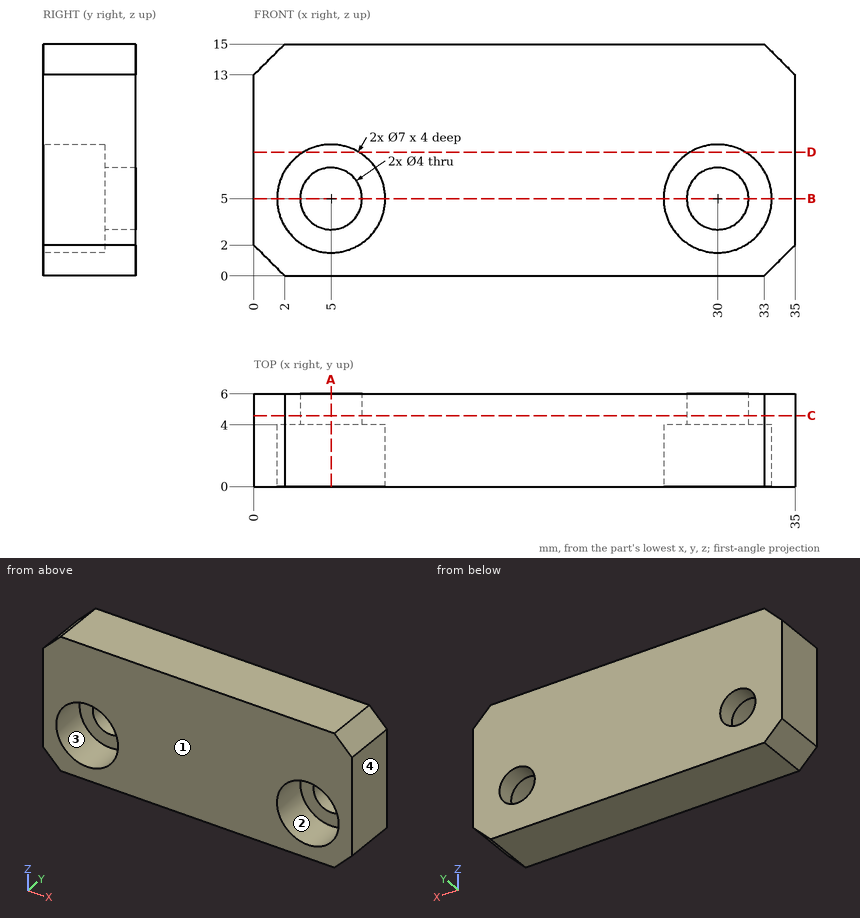
Could you check a few things on this drawing? It's one solid part, dimensions in mm from its lowest x, y, z. Coordinates: 2 decimals unless noted, no trailing zeros. Order: outer loops, then holes, each group sorted by start corner. A loop starts at its lowest first (then second) coordinate and runs counter-clockwise, first axis right, second up.
1. If we section it at C-C (y = 4.6): Please give me the cut outline in (x, z), then the cut area to 3 significant figures.
2. I need wall thicknesses on line 1 (X direction, y = 2.2, z = 4.5); line 2 (Z direction, x = 5, y = 1.15); line 3 (Z direction, x = 30, y = 4.85). Which ranges of each line are inside material? Lowest first, please.
3. If we section it at D-D (z = 8): Please give me the cut outline in (x, y), then the cut area to 3 significant figures.
4. If we section it at A-A (x = 5): Please give me the cut outline in (y, z).
5. If we section it at B-B (z = 5): Please give me the cut outline in (x, y).
6. Thinking about a two-plate mould opening in X: for the marked faces 1, 2, 3 and 4, which applies, +X half, -X half, draft (parallel to the pull), parting line (faces both ways), or undercut?
7. I'm going to push flat-ended pins straight in: pin 1 (5.5 mm diameter, centred on x = 30, z = 5, fed in from -Y); pin 2 (7.5 mm diameter, centred on x = 5, z = 4, fed in from -Y); pin 3 (3.5 mm diameter, centred on x = 5, z = 5, fed in from +Y). Where does each tip first touch, or does it pass through?
Entries:
1. outline: (0, 2) - (2, 0) - (33, 0) - (35, 2) - (35, 13) - (33, 15) - (2, 15) - (0, 13) - close; hole circle Ø4 at (5, 5); hole circle Ø4 at (30, 5)
1. area: 492 mm2
2. line 1: x = 0 to 1.54, 8.46 to 26.54, 33.46 to 35
2. line 2: z = 0 to 1.5, 8.5 to 15
2. line 3: z = 0 to 3, 7 to 15
3. outline: (0, 0) - (3.2, 0) - (3.2, 4) - (6.8, 4) - (6.8, 0) - (28.2, 0) - (28.2, 4) - (31.8, 4) - (31.8, 0) - (35, 0) - (35, 6) - (0, 6) - close
3. area: 181 mm2
4. outline: (0, 0) - (6, 0) - (6, 3) - (4, 3) - (4, 1.5) - (0, 1.5) - close; (0, 8.5) - (4, 8.5) - (4, 7) - (6, 7) - (6, 15) - (0, 15) - close
5. outline: (0, 0) - (1.5, 0) - (1.5, 4) - (3, 4) - (3, 6) - (0, 6) - close; (7, 4) - (8.5, 4) - (8.5, 0) - (26.5, 0) - (26.5, 4) - (28, 4) - (28, 6) - (7, 6) - close; (32, 4) - (33.5, 4) - (33.5, 0) - (35, 0) - (35, 6) - (32, 6) - close
6. face 1: draft
6. face 2: undercut
6. face 3: undercut
6. face 4: +X half
7. pin 1: stops at y = 4
7. pin 2: stops at y = 0
7. pin 3: passes through
